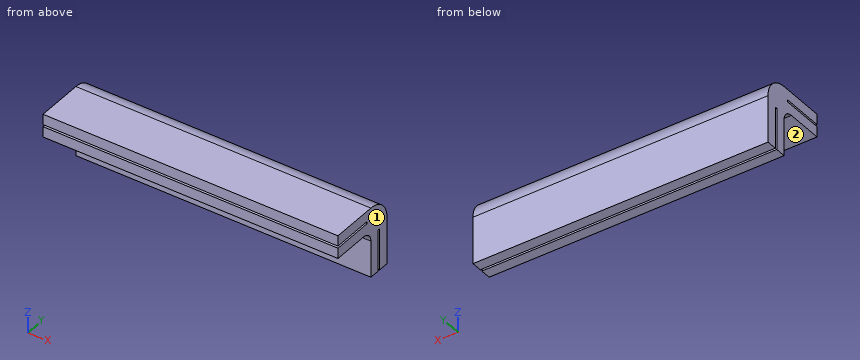
from build123d import *

# Parameters (mm, degrees)
BOSS_EXTRUDE1_DEPTH      = 141
BOSS_EXTRUDE1_DEPTH_BACK = 141
CAVITY1_START            = -2
CAVITY1_OUTLINE_W        = 282
CAVITY1_OUTLINE_H        = 40
CAVITY1_DEPTH            = 2


# Read off the part's stored shape, not the designer's step: Cavity1
with BuildPart() as part:
    # Sketch2 → Boss-Extrude1 (new, two sides: drawn at the far end of the back side and taken through both)
    with BuildSketch(Plane(origin=(0, 0, 0), x_dir=(0, 0, -1), z_dir=(1, 0, 0)).offset(-BOSS_EXTRUDE1_DEPTH_BACK)):
        with BuildLine():
            Line((12, 220), (12, 185))
            Line((12, 185), (-10, 185))
            Line((-10, 185), (-10, 230))
            ThreePointArc((-10, 230), (-3.556349186, 245.556349186), (12, 252))
            Line((12, 252), (57, 252))
            Line((57, 252), (57, 242))
            Line((57, 242), (17, 242))
            Line((17, 242), (17, 240))
            Line((17, 240), (57, 240))
            Line((57, 240), (57, 230))
            Line((57, 230), (22, 230))
            ThreePointArc((22, 230), (14.928932188, 227.071067812), (12, 220))
        make_face()
    extrude(amount=BOSS_EXTRUDE1_DEPTH + BOSS_EXTRUDE1_DEPTH_BACK)

    # Cavity1 outline → Cavity1 (cut)
    with BuildSketch(Plane.XY.offset(CAVITY1_START)):
        with Locations((0, 205)):
            Rectangle(CAVITY1_OUTLINE_W, CAVITY1_OUTLINE_H)
    extrude(amount=CAVITY1_DEPTH, mode=Mode.SUBTRACT)


solid = part.part
Geometry: final body of the model. Coordinates: model frame, mm. Face numbers are marked on the shaded views. A direction names the side the tool comes from. Give positions to 0.01 mm unless a question says otherwise; leave off trailing zeros. Write each loop counter-clockwise with the first axis right and the second up, starting at its lowest first coordinate (ties: lowest second). Pieces come first, ordered by that corner, then holes. Notation, with made-up numbers: (89.25, -32.75) -> (125.25, -32.75) arc R24 cw to (125.25, -7.75) -> close; hole circle Ø9 at (16, 64.25). An arc over 180 degrees is marked (long way). Answer as a JSON object with one key per item and string values.
1. Cut plane A-A on y = 201.5. Output: boundary loops of the cut face in (x, z), and give its area (3 significant figures).
Ans:
{"outline": "(-141, -12) -> (141, -12) -> (141, -2) -> (-141, -2) -> close; (-141, 0) -> (141, 0) -> (141, 10) -> (-141, 10) -> close", "area": "5,640 mm^2"}
2. Access query for the marked faces 1 and 2. Directions: +Z, -Z, +X, -X, +Y, -Y. A direction counts if a zero-diameter tool reaches every point of the face in a straight line with its end or side. Return the directions, or none.
Ans:
{"face 1": "+Z, -Z, +X, +Y, -Y", "face 2": "-Z, +X, -X, -Y"}
3. Cut plane C-C on x = -13. Output: boundary loops of the cut face in (y, z).
Ans:
{"outline": "(185, -12) -> (220, -12) arc R10 cw to (230, -22) -> (230, -57) -> (240, -57) -> (240, -17) -> (242, -17) -> (242, -57) -> (252, -57) -> (252, -12) arc R22 ccw to (230, 10) -> (185, 10) -> (185, 0) -> (225, 0) -> (225, -2) -> (185, -2) -> close"}
4. Cut plane B-B on z = -27. Output: boundary loops of the cut face in (x, y), and give its area (3 significant figures).
Ans:
{"outline": "(-141, 230) -> (141, 230) -> (141, 240) -> (-141, 240) -> close; (-141, 242) -> (141, 242) -> (141, 252) -> (-141, 252) -> close", "area": "5,640 mm^2"}
5. Contact query for flat-ended pins moving along their axis: pin 1 (3 mm diameter, centred on x = -74, z = -19.5, fed in from -Y); pin 2 (20 mm diameter, centred on x = -69.5, y = 196.5, fed in from -Z); pin 3 (17.5 mm diameter, centred on x = 48.5, z = -31.5, fed in from -Y). Output: stop coordinate, or through.
Ans:
{"pin 1": "stops at y = 229.17", "pin 2": "stops at z = -12", "pin 3": "stops at y = 230"}
6. Ray query, probe 1 along Y at (x, z) = (-90, -35.5); probe 2 along Z at (x, y) = (-7, 198); probe 3 along Z at (x, y) = (94, 223). Return the intervals inside material, ascending. Write a range as from..to.
Ans:
{"probe 1": "y = 230..240, 242..252", "probe 2": "z = -12..-2, 0..10", "probe 3": "z = -12.46..-2, 0..10"}
